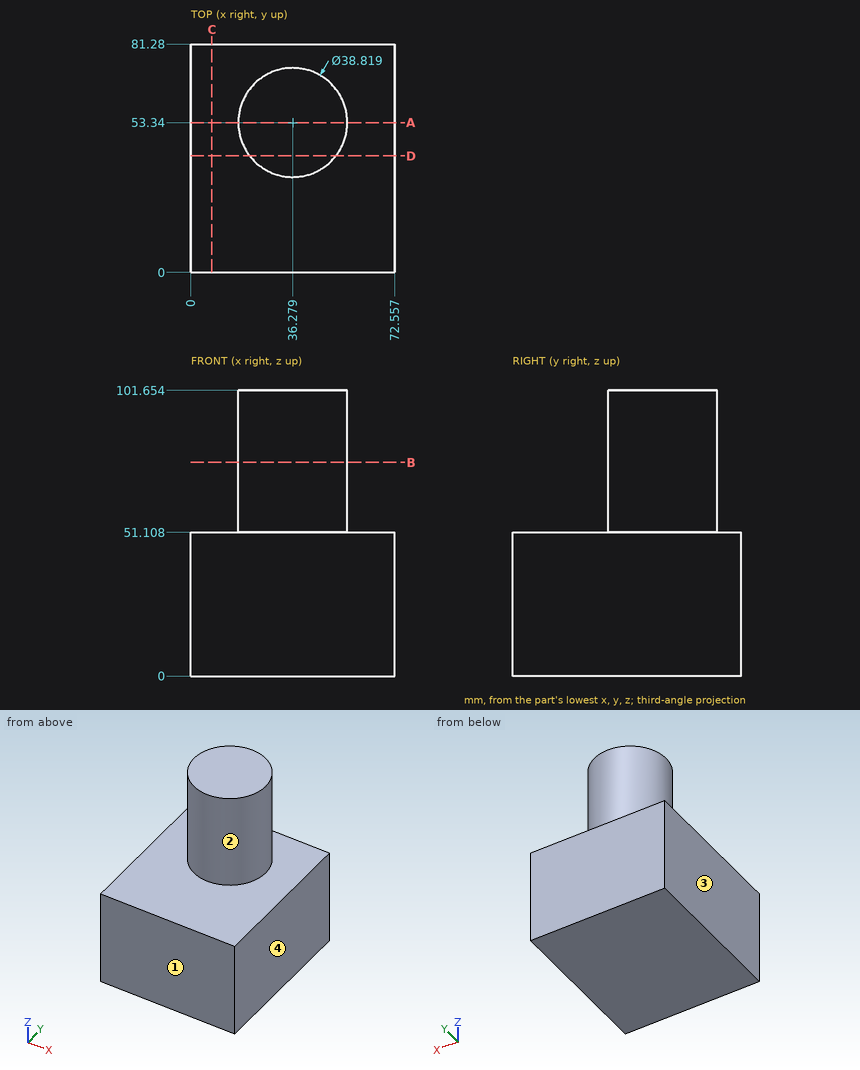
Design review of the part shown in the three views and the two pictorial views. Dimensions are in mm from the part's minimum x, y and z. Coordinates: 2 decimals unless noted, no trailing zeros. Loops run counter-clockwise (first coordinate to the right, second up) from the corner with the lowest first, then second, coordinate; pieces in that order, holes last. Notation, with made-up numbers: M 73,-1 L 113,-1 A17 cw 113,8 Z; hole C 17.25,74 d7. An arc over 180 degrees is marked long. One line per question, with ' | ' between items.
(1) We need section A-A (y = 53.34). Give the boundary of the cut face in (x, z) (1 decimal), and give its area (3 significant figures).
Filled in:
outline: M 0,0 L 72.6,0 L 72.6,51.1 L 55.7,51.1 L 55.7,101.7 L 16.9,101.7 L 16.9,51.1 L 0,51.1 Z | area: 5,670 mm^2
(2) We need section B-B (z = 76). Give the boundary of the cut face in (x, y).
Filled in:
outline: C 36.28,53.34 d38.82
(3) We need section D-D (y = 41.5). Give the boundary of the cut face in (x, z) (1 decimal), and give its area (3 significant figures).
Filled in:
outline: M 0,0 L 72.6,0 L 72.6,51.1 L 51.7,51.1 L 51.7,101.7 L 20.9,101.7 L 20.9,51.1 L 0,51.1 Z | area: 5,260 mm^2
(4) For pin 1 Ø2 at (x, z) = (34, 59.5) entering from +Y; pin 2 Ø1 at (x, y) = (64.5, 31) entering from +Z; pin 3 Ø5 at (y, z) = (50.5, 56) entering from -X, all flat-tipped, find the tip position at first contact; note any pin that passes through.
Filled in:
pin 1: stops at y = 72.71 | pin 2: stops at z = 51.11 | pin 3: stops at x = 16.87
(5) Wall thickness on probe 1 along Z at (x, y) = (48, 20); probe 2 along X at (y, z) = (54, 91.5); probe 3 along X at (y, z) = (50.5, 74.5): over which ranges is each line inside the solid? List them lowest first.
Filled in:
probe 1: z = 0 to 51.11 | probe 2: x = 16.88 to 55.68 | probe 3: x = 17.08 to 55.48
(6) Draft analysis for pull direction X (two halves, no side actions). For the marked faces 1, 2, 3 and 4, state which applies: released by +X, released by -X, zero draft, split by the parting line, or undercut.
Filled in:
face 1: zero draft | face 2: split by the parting line | face 3: released by -X | face 4: released by +X
(7) We need section C-C (x = 7.5). Give the boundary of the cut face in (y, z), and give its area (3 significant figures).
Filled in:
outline: M 0,0 L 81.28,0 L 81.28,51.11 L 0,51.11 Z | area: 4,150 mm^2
